Build history of the part. All positions in model axes, mm. A direction names the side the tool comes from. Coordinates: 2 decimals unless noted, no trailing zeros. Order: outer loops, then holes, each group sorted by start corner. A loop starts at its lowest first (then second) coordinate and runs counter-clockwise, first axis right, second up. Notation, with made-up numbers: (-8.5, 39) - (-4.5, 39) arc R37 cw to (-4.5, 76) - close; hole circle Ø11 at (-25.5, 29.5). An arc over 180 degrees is marked (long way). Write each question's results on one line, items separated by ' | '.
from build123d import *

# Parameters (mm, degrees)
F0_W          = 85
F0_H          = 38
F1_DEPTH      = 27.5
F2_W          = 65
F2_H          = 30
F3_DEPTH      = 27.501
F3_DEPTH_BACK = 27.501
F4_W          = 5
F4_H          = 18
F5_DEPTH      = 27.501
F5_DEPTH_BACK = 27.501
F7_DEPTH      = 38.001


with BuildPart() as f1:
    # F0 (on Front) → F1 (new body, symmetric)
    with BuildSketch(Plane.XZ):
        with Locations((-42.5, 19)):
            Rectangle(F0_W, F0_H)
    extrude(amount=F1_DEPTH, both=True)

    # F2 (on Front) → F3 (cut, two sides)
    with BuildSketch(Plane.XZ) as f3_sk:
        with Locations((-52.5, 23)):
            Rectangle(F2_W, F2_H)
    extrude(amount=-F3_DEPTH, mode=Mode.SUBTRACT)
    extrude(f3_sk.sketch, amount=F3_DEPTH_BACK, mode=Mode.SUBTRACT)

    # F4 (on Front) → F5 (cut, two sides)
    with BuildSketch(Plane.XZ) as f5_sk:
        with Locations((-2.5, 24)):
            Rectangle(F4_W, F4_H)
    extrude(amount=F5_DEPTH, mode=Mode.SUBTRACT)
    extrude(f5_sk.sketch, amount=-F5_DEPTH_BACK, mode=Mode.SUBTRACT)

    # F6 (on Top) → F7 (cut, through all)
    with BuildSketch(Plane.XY):
        with BuildLine():
            Line((-4.5, 10), (-6, 10))
            Line((-6, 10), (-6, 9.5))
            ThreePointArc((-6, 9.5), (-5.290569415, 9.8717082451), (-4.5, 10))
        make_face()
        with BuildLine():
            Line((4.5, 10), (-4.5, 10))
            ThreePointArc((-4.5, 10), (-5.290569415, 9.8717082451), (-6, 9.5))
            Line((-6, 9.5), (-6, 5.5))
            ThreePointArc((-6, 5.5), (-5.290569415, 5.1282917549), (-4.5, 5))
            Line((-4.5, 5), (4.5, 5))
            ThreePointArc((4.5, 5), (5.290569415, 5.1282917549), (6, 5.5))
            Line((6, 5.5), (6, 9.5))
            ThreePointArc((6, 9.5), (5.290569415, 9.8717082451), (4.5, 10))
        make_face()
        with BuildLine():
            Line((-6, 5.5), (-6, 9.5))
            ThreePointArc((-6, 9.5), (-7, 7.5), (-6, 5.5))
        make_face()
        with BuildLine():
            Line((6, 10), (4.5, 10))
            ThreePointArc((4.5, 10), (5.290569415, 9.8717082451), (6, 9.5))
            Line((6, 9.5), (6, 10))
        make_face()
        with BuildLine():
            ThreePointArc((-4.5, 5), (-5.290569415, 5.1282917549), (-6, 5.5))
            Line((-6, 5.5), (-6, -5.5))
            ThreePointArc((-6, -5.5), (-6.8717082451, -8.290569415), (-4.5, -10))
            Line((-4.5, -10), (4.5, -10))
            ThreePointArc((4.5, -10), (6.8717082451, -8.290569415), (6, -5.5))
            Line((6, -5.5), (6, 5.5))
            ThreePointArc((6, 5.5), (5.290569415, 5.1282917549), (4.5, 5))
            Line((4.5, 5), (-4.5, 5))
        make_face()
        with BuildLine():
            ThreePointArc((6, 5.5), (7, 7.5), (6, 9.5))
            Line((6, 9.5), (6, 5.5))
        make_face()
    extrude(amount=F7_DEPTH, mode=Mode.SUBTRACT)


solid = f1.part
1. Band-saw the part on A-A on z = 11. Give the cut face in (x, y).
Solved:
outline: (-20, -27.5) - (0, -27.5) - (0, -10) - (-4.5, -10) arc R2.5 cw to (-6, -5.5) - (-6, 5.5) arc R2.5 cw to (-6, 9.5) - (-6, 10) - (0, 10) - (0, 27.5) - (-20, 27.5) - close
2. Band-saw the part on B-B on y = 22.5. Give the cut face in (x, z).
Solved:
outline: (-85, 0) - (0, 0) - (0, 15) - (-5, 15) - (-5, 33) - (0, 33) - (0, 38) - (-20, 38) - (-20, 8) - (-85, 8) - close
3. Drop flat-ended pins along their axis: pin 1 Ø2 at (x, y) = (-53.5, 13.5) entering from +Z; pin 2 Ø5.5 at (y, z) = (2.5, 11) entering from +X; pin 3 Ø1 at (y, z) = (-18.5, 15) entering from -X. Give the stop position or say it passes through.
Solved:
pin 1: stops at z = 8 | pin 2: stops at x = -6 | pin 3: stops at x = -20
4. Probe line 1 (Z direction, x = -70, y = 9); line 2 (X direction, y = 23, z = 34.5); line 3 (X direction, y = -23, z = 25.5). List the from-to ranges inside material, lowest first.
Solved:
line 1: z = 0 to 8 | line 2: x = -20 to 0 | line 3: x = -20 to -5
5. Band-saw the part on D-D on x = -76.5. Give the cut face in (y, z).
Solved:
outline: (-27.5, 0) - (27.5, 0) - (27.5, 8) - (-27.5, 8) - close
6. Band-saw the part on C-C on z = 25. Give the cut face in (x, y), then the cut area to 3 significant figures.
Solved:
outline: (-20, -27.5) - (-5, -27.5) - (-5, -9.95) arc R2.5 cw to (-6, -5.5) - (-6, 5.5) arc R2.5 cw to (-6, 9.5) - (-6, 10) - (-5, 10) - (-5, 27.5) - (-20, 27.5) - close | area: 800 mm2
7. Tool access for faces 1 (the face through (-53, 0, 8)), 2 (the face through (-3, 10, 14.5)), 3 (the face through (-3, -19, 33)): list every direction of +Z, -Z, +X, -X, +Y, -Y with a clear straight run to the whole face (end or side of a thin tool).
Solved:
face 1: +Z, -X, +Y, -Y | face 2: +Z, -Z, +X | face 3: +X, +Y, -Y
